```python
from build123d import *

# Parameters (mm, degrees)
SKETCH1_R           = 5.08
SKETCH1_R_2         = 1.778
BOSS_EXTRUDE1_DEPTH = 10.16
FILLET1_R           = 2.54
SKETCH2_W           = 7.62
SKETCH2_H           = 7.62
BOSS_EXTRUDE3_DEPTH = 6.35


with BuildPart() as part:
    # Sketch1 → Boss-Extrude1 (new body)
    with BuildSketch(Plane.XY):
        with BuildLine():
            Line((-6.35, 12.7), (-6.35, 10.998522628))
            ThreePointArc((-6.35, 10.998522628), (0, -12.7), (6.35, 10.998522628))
            Line((6.35, 10.998522628), (6.35, 12.7))
            Line((6.35, 12.7), (-6.35, 12.7))
        make_face()
        Circle(SKETCH1_R, mode=Mode.SUBTRACT)
        with Locations((0, 8.128)):
            Circle(SKETCH1_R_2, mode=Mode.SUBTRACT)
        with Locations((8.128, 0)):
            Circle(SKETCH1_R_2, mode=Mode.SUBTRACT)
        with Locations((0, -8.128)):
            Circle(SKETCH1_R_2, mode=Mode.SUBTRACT)
        with Locations((-8.128, 0)):
            Circle(SKETCH1_R_2, mode=Mode.SUBTRACT)
    extrude(amount=BOSS_EXTRUDE1_DEPTH)

    # Fillet1
    fillet1_edges = [part.edges().sort_by_distance(p)[0] for p in [
        (-6.35, 10.998522628, 5.08),
        (6.35, 10.998522628, 5.08),
    ]]
    fillet(fillet1_edges, radius=FILLET1_R)

    # Sketch2 → Boss-Extrude3 (add)
    with BuildSketch(Plane(origin=(0, 12.7, 0), x_dir=(1, 0, 0), z_dir=(0, 1, 0))):
        with Locations((0, -5.08)):
            Rectangle(SKETCH2_W, SKETCH2_H)
    extrude(amount=BOSS_EXTRUDE3_DEPTH)


solid = part.part
```
CAD build for the part. Positions are in the model's coordinates, mm. A direction names the side the tool comes from. Coordinates: 2 decimals unless noted, no trailing zeros. Order: outer loops, then holes, each group sorted by start corner. A loop starts at its lowest first (then second) coordinate and runs counter-clockwise, first axis right, second up. Notation, with made-up numbers: (38.25, 40.25) -> (52.25, 40.25) arc R24 ccw to (52.25, 51.25) -> close; hole circle Ø7 at (47.5, -6.5). An arc over 180 degrees is marked (long way). Use one line per item in the form item = value. Start each with the question number.
1) Tool access for faces 5 (the flat face through (-3.81, 16, 5)), 6 (the flat face through (0, 16, 1.27)), 7 (the flat face through (0, 16, 8.89)), 8 (the flat face through (0, 19.05, 5)), 9 (the cylindrical face through (-0.23, 9.89, 5.01)): list every direction of +Z, -Z, +X, -X, +Y, -Y with a clear straight run to the whole face (end or side of a thin tool).
2) Band-saw the part on C-C on x = 8. Give the cut face in (y, z).
3) Drop flat-ended pins along their axis: pin 1 (5 mm diameter, centred on y = 16, z = 4.5, fed in from +X); pin 2 (3 mm diameter, centred on x = 1, y = 17, fed in from +Z); pin 3 (4 mm diameter, centred on y = -3, z = 6, fed in from -X). Give the stop position or say it passes through.
4) Band-saw the part on A-A on y = 0. Give the cut face in (x, z).
5) Band-saw the part on D-D on y = -7. Give the cut face in (x, z), then the cut area to 3 significant figures.
6) Pull direction X, two halves, no side cores. Call faces 1 (the flat face through (-4, 12.7, 5)), 2 (the cylindrical face through (-6.622, 11.234, 5.151)), 3 (the cylindrical face through (6.35, 0.08, 5.01)), 4 (the flat face through (3.81, 16, 5)): +X half, -X half, draft (parallel to the pull), parting line (faces both ways), or undercut.
7) Band-saw the part on B-B on x = 0. Give the cut face in (y, z), then the cut area to 3 significant figures.
8) Drill centre lines: L1, parallel to Y at x = 7.5, z = 4.75; L2, parallel to X at y = -1, z = 2.75; L3, parallel to Y at x = -1.5, z = 1. Where is each one in solid material? Low to high. Write a range as [from, to].
Entries:
q1.face_5 = +Z, -Z, -X, +Y
q1.face_6 = -Z, +X, -X, +Y
q1.face_7 = +Z, +X, -X, +Y
q1.face_8 = +Z, -Z, +X, -X, +Y
q1.face_9 = +Z, -Z
q2.outline = (-9.86, 0) -> (-1.77, 0) -> (-1.77, 10.16) -> (-9.86, 10.16) -> close; (1.77, 0) -> (9.86, 0) -> (9.86, 10.16) -> (1.77, 10.16) -> close
q3.pin_1 = 3.81
q3.pin_2 = 8.89
q3.pin_3 = -12.66
q4.outline = (-12.7, 0) -> (-9.91, 0) -> (-9.91, 10.16) -> (-12.7, 10.16) -> close; (-6.35, 0) -> (-5.08, 0) -> (-5.08, 10.16) -> (-6.35, 10.16) -> close; (5.08, 0) -> (6.35, 0) -> (6.35, 10.16) -> (5.08, 10.16) -> close; (9.91, 0) -> (12.7, 0) -> (12.7, 10.16) -> (9.91, 10.16) -> close
q5.outline = (-10.6, 0) -> (-1.37, 0) -> (-1.37, 10.16) -> (-10.6, 10.16) -> close; (1.37, 0) -> (10.6, 0) -> (10.6, 10.16) -> (1.37, 10.16) -> close
q5.area = 187 mm2
q6.face_1 = draft
q6.face_2 = -X half
q6.face_3 = undercut
q6.face_4 = +X half
q7.outline = (-12.7, 0) -> (-9.91, 0) -> (-9.91, 10.16) -> (-12.7, 10.16) -> close; (-6.35, 0) -> (-5.08, 0) -> (-5.08, 10.16) -> (-6.35, 10.16) -> close; (5.08, 0) -> (6.35, 0) -> (6.35, 10.16) -> (5.08, 10.16) -> close; (9.91, 0) -> (12.7, 0) -> (12.7, 1.27) -> (19.05, 1.27) -> (19.05, 8.89) -> (12.7, 8.89) -> (12.7, 10.16) -> (9.91, 10.16) -> close
q7.area = 131 mm2
q8.L1 = [-10.25, -1.66], [1.66, 10.25]
q8.L2 = [-12.66, -9.6], [-6.66, -4.98], [4.98, 6.66], [9.6, 12.66]
q8.L3 = [-12.61, -9.08], [-7.17, -4.85], [4.85, 7.17], [9.08, 12.7]
